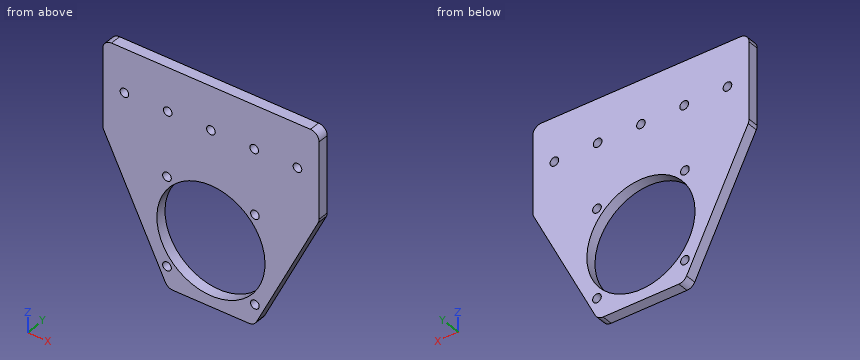
from build123d import *

# Parameters (mm, degrees)
SKETCH1_R             = 15.875
SKETCH1_R_2           = 1.27
INITIAL_BRACKET_DEPTH = 3.175
EDGE_FILLET_R         = 2.54
LPATTERN1_OUTLINE_R   = 1.27
LPATTERN1_DEPTH       = 3.175


# Read off the part's stored shape, not the designer's step: LPattern1
with BuildPart() as part:
    # Sketch1 → Initial Bracket (new body)
    with BuildSketch(Plane(origin=(0, 0, 0), x_dir=(1, 0, 0), z_dir=(0, 1, 0))):
        Polygon((-31.75, -31.75), (31.75, -31.75), (31.75, -6.35), (12.7, 31.75), (-12.7, 31.75), (-31.75, -6.35), align=None)
        with Locations(Location((0, 12.7, 0), (0, 0, 270))):
            Circle(SKETCH1_R, mode=Mode.SUBTRACT)
        with Locations(Location((12.909118174, 25.609118174, 0), (0, 0, 270))):
            Circle(SKETCH1_R_2, mode=Mode.SUBTRACT)
        with Locations(Location((12.909118174, -0.209118174, 0), (0, 0, 270))):
            Circle(SKETCH1_R_2, mode=Mode.SUBTRACT)
        with Locations(Location((-12.909118174, -0.209118174, 0), (0, 0, 270))):
            Circle(SKETCH1_R_2, mode=Mode.SUBTRACT)
        with Locations(Location((-12.909118174, 25.609118174, 0), (0, 0, 270))):
            Circle(SKETCH1_R_2, mode=Mode.SUBTRACT)
        with Locations(Location((-25.4, -19.05, 0), (0, 0, 270))):
            Circle(SKETCH1_R_2, mode=Mode.SUBTRACT)
    extrude(amount=INITIAL_BRACKET_DEPTH)

    # Edge Fillet
    edge_fillet_edges = [part.edges().sort_by_distance(p)[0] for p in [
        (31.75, 1.5875, 31.75),
        (-31.75, 1.5875, 31.75),
        (-31.75, 1.5875, 6.35),
        (-12.7, 1.5875, -31.75),
        (12.7, 1.5875, -31.75),
        (31.75, 1.5875, 6.35),
    ]]
    fillet(edge_fillet_edges, radius=EDGE_FILLET_R)

    # LPattern1 outline → LPattern1 (cut)
    with BuildSketch(Plane(origin=(0, 0, 0), x_dir=(1, 0, 0), z_dir=(0, 1, 0))):
        with Locations((25.4, -19.05)):
            Circle(LPATTERN1_OUTLINE_R)
        with Locations((12.7, -19.05)):
            Circle(LPATTERN1_OUTLINE_R)
        with Locations((0, -19.05)):
            Circle(LPATTERN1_OUTLINE_R)
        with Locations((-12.7, -19.05)):
            Circle(LPATTERN1_OUTLINE_R)
    extrude(amount=LPATTERN1_DEPTH, mode=Mode.SUBTRACT)


solid = part.part
Can you work these out from the model? Positions are in its coordinate system, mm. Give positions to 0.01 mm unless a question says otherwise; leave off trailing zeros. Loops run counter-clockwise (first coordinate to the right, second up) from the corner with the lowest first, then second, coordinate; pieces in that order, holes last. Notation, with made-up numbers: M 65,56.5 L 116,56.5 A24 cw 116,85.5 Z; hole C 18.25,55 d8. An arc over 180 degrees is marked long. One line per item, written item: value.
1) Imagine slicing it at C-C on z = -12.7. Write out the boundary of the cut face in (x, y) (3 decimals), and give its area (3 significant figures).
Geometry check:
outline: M -22.225,0 L -15.875,0 L -15.875,3.175 L -22.225,3.175 Z; M 15.875,0 L 22.225,0 L 22.225,3.175 L 15.875,3.175 Z
area: 40.3 mm²
2) Imagine slicing it at B-B on x = 25.4. Write out the boundary of the cut face in (y, z) (3 decimals).
Geometry check:
outline: M 0,-6.35 L 3.175,-6.35 L 3.175,17.78 L 0,17.78 Z; M 0,20.32 L 3.175,20.32 L 3.175,31.75 L 0,31.75 Z
3) Please list where these lines run through material, in increasing order: line 1 (X direction, y = 1.7, z = 19.05); line 2 (X direction, y = 2.7, z = 0) (3 decimals); line 3 (Z direction, x = 1.5, y = 2.9).
Geometry check:
line 1: x = -31.75 to -26.67, -24.13 to -13.97, -11.43 to -1.27, 1.27 to 11.43, 13.97 to 24.13, 26.67 to 31.75
line 2: x = -28.575 to -14.162, -11.656 to -9.525, 9.525 to 11.656, 14.162 to 28.575
line 3: z = -31.75 to -28.5, 3.1 to 31.75
4) Imagine slicing it at D-D on y = 1.8. Count the separate pieces of the cut face and the enclosed holes in it, and give its area (3 significant figures).
Geometry check:
separate pieces: 1
enclosed holes: 10
area: 2,470 mm²
5) I'm going to push flat-ended pins straight in: pin 1 (3 mm diameter, centred on x = -12.7, z = 19.05, fed in from -Y); pin 2 (2 mm diameter, centred on x = -12.91, z = -25.61, fed in from -Y); pin 3 (1.5 mm diameter, centred on x = 19, y = 0.5, fed in from -Z). Where does each tip first touch, or does it pass through?
Geometry check:
pin 1: stops at y = 0
pin 2: passes through
pin 3: stops at z = -20.65
6) Imagine slicing it at A-A on z = 19.05. Write out the boundary of the cut face in (x, y) (3 decimals).
Geometry check:
outline: M -31.75,0 L -26.67,0 L -26.67,3.175 L -31.75,3.175 Z; M -24.13,0 L -13.97,0 L -13.97,3.175 L -24.13,3.175 Z; M -11.43,0 L -1.27,0 L -1.27,3.175 L -11.43,3.175 Z; M 1.27,0 L 11.43,0 L 11.43,3.175 L 1.27,3.175 Z; M 13.97,0 L 24.13,0 L 24.13,3.175 L 13.97,3.175 Z; M 26.67,0 L 31.75,0 L 31.75,3.175 L 26.67,3.175 Z
